Autodesk Inventor part; units mm, degrees
ref_plane "YZ Plane" through (0, 0, 0) normal (1, 0, 0) x (0, 1, 0)
ref_plane "XZ Plane" through (0, 0, 0) normal (0, 1, 0) x (-1, 0, 0)
ref_plane "XY Plane" through (0, 0, 0) normal (0, 0, 1) x (1, 0, 0)
sketch "Sketch1" plane through (0, 0, 0) normal (0, 0, 1) x (1, 0, 0)
  line L0 (0, 0) -> (35, 0)
  line L1 (35, 0) -> (35, 12)
  line L2 (0, 12) -> (0, 0)
  line L3 (0, 12) -> (-0.0372, 12)
  line L4 (35.0398, 12) -> (35, 12)
  line L5 (-0.0372, 12) -> (-0.0372, 30)
  line L6 (35.0398, 12) -> (35.0398, 30)
  arc A0 (35.0398, 30) -> (-0.0372, 30) centre (17.5013, 30) ccw
  circle A1 centre (17.5013, 30) radius 2
  dimension "d0" = 35
  dimension "d1" = 12
  dimension "d4" = 18
  dimension "d6" = 4
extrude "Extrusion1" add sketch "Sketch1" along normal blind 22.5
sketch "Sketch2" plane through (0, 0, 22.5) normal (0, 0, 1) x (1, 0, 0)
  line L0 (0, 2) -> (35, 2)
  line L1 (35, 2) -> (35, 10)
  line L2 (35, 10) -> (0, 10)
  line L3 (0, 10) -> (0, 2)
  point P0 (0, 0)
extrude "Extrusion2" cut sketch "Sketch2" against normal blind 20
sketch "Sketch3" plane through (-0.0372, 12, 0) normal (-1, 0, 0) x (0, 0, 1)
  point P0 (0, -12)
ref_plane "Work Plane1" through (17.5013, 47.5385, 0) normal (0, -1, 0) x (1, 0, 0)
sketch "Sketch4" plane through (17.5013, 47.5385, 0) normal (0, -1, 0) x (1, 0, 0)
  line L0 (17.5385, 0) -> (17.5385, 22.5)
  line L1 (-17.5385, 0) -> (-17.5385, 22.5)
  line L2 (17.5385, 20.5) -> (-17.5385, 20.5)
  line L3 (-17.5385, 20.5) -> (-17.5385, 2)
  line L4 (-17.5385, 2) -> (17.5385, 2)
  line L5 (17.5385, 2) -> (17.5385, 20.5)
  line L6 (17.5385, 22.5) -> (-17.5385, 22.5)
  point P0 (-17.5013, 0)
  dimension "d11" = 18.5
  dimension "d12" = 2
extrude "Extrusion3" cut sketch "Sketch4" along normal blind 35.5 contours L4 L1 L2 L0
properties part number "Maintients poullies V4"
The listing builds one solid part. Answer for the finished solid, in the listing's coordinates (mm). A direction names the side the tool comes from. Give positions to 0.01 mm unless a question says otherwise; leave off trailing zeros. Write each loop counter-clockwise with the first axis right and the second up, starting at its lowest first coordinate (ties: lowest second). Pieces come first, ordered by that corner, then holes. Notation, with made-up numbers: (-1, -31) - (42, -31) arc R31 ccw to (42, -3) - close; hole circle Ø3 at (49, 62.25). An arc over 180 degrees is marked (long way). One line per question, with ' | ' between items. Start each with the question number.
1. Given P1, Ø5.5, axis at x = 21, z = 14, coming from the +Y side; P2, Ø6, axis at y = 7.5, z = 14, coming from the -X side; P3, Ø2.5, axis at x = 24.5, y = 7.5, coming from the +Z side; P4, Ø3.5, axis at x = 17.5, y = 30, coming from the -Z side, each flat-ended and moving along its own axis, determine where each tip first touches the part or whether it passes through.
2. Determine the mould class of faces 6 (the face through (18.424, 31.774, 21.486)), 7 (the face through (17, 0, 11)), 8 (the face through (17, 6, 2.5)), 9 (the face through (-0.037, 20, 21)) for opening direction Y: +Y half, -Y half, draft (parallel to the pull), parting line (faces both ways), or undercut.
3. Section D-D, the plane x = 24 is taken. Determine the outline of the cut face in (y, z), then the cut area to 3 significant figures.
4. Section B-B, the plane x = 7.5 is taken. Determine the outline of the cut face in (y, z), then the cut area to 3 significant figures.
5. For faces 1 (the face through (17.116, 47.534, 0.986)), 2 (the face through (35, 1, 9)), 3 (the face through (18, 26, 20.5)), 4 (the face through (35.04, 20, 21)), 5 (the face through (17, 2, 13)), determine the directions among +Z, -Z, +X, -X, +Y, -Y from which every point of the face is accessible in a straight line to the end or side of a thin tool.
6. Section A-A, the plane y = 20 is taken. Determine the outline of the cut face in (x, z), then the cut area to 3 significant figures.
7. Section C-C, the plane y = 44 is taken. Determine the outline of the cut face in (x, z).
8. Straight lines are drawn through the part: line 1 (Y direction, x = 19.5, z = 20); line 2 (Z direction, x = 32.5, y = 21.5); line 3 (X direction, y = 30, z = 20.9). For each, find the intervals that lie inside material, in ascending order.
Result:
1) P1: stops at y = 12.04 | P2: stops at x = 0 | P3: stops at z = 2.5 | P4: passes through
2) face 6: undercut | face 7: -Y half | face 8: undercut | face 9: draft
3) outline: (0, 0) - (46.29, 0) - (46.29, 2) - (12.04, 2) - (12.04, 20.5) - (46.29, 20.5) - (46.29, 22.5) - (10, 22.5) - (10, 2.5) - (2, 2.5) - (2, 22.5) - (0, 22.5) - close | area: 248 mm2
4) outline: (0, 0) - (44.41, 0) - (44.41, 2) - (12.04, 2) - (12.04, 20.5) - (44.41, 20.5) - (44.41, 22.5) - (10, 22.5) - (10, 2.5) - (2, 2.5) - (2, 22.5) - (0, 22.5) - close | area: 240 mm2
5) face 1: +Z, -Z, +Y | face 2: +Z, -Z, +X, -Y | face 3: +X, -X, +Y | face 4: +Z, -Z, +X, +Y, -Y | face 5: +Z, +X, -X
6) outline: (-0.04, 0) - (35.04, 0) - (35.04, 2) - (-0.04, 2) - close; (-0.04, 20.5) - (35.04, 20.5) - (35.04, 22.5) - (-0.04, 22.5) - close | area: 140 mm2
7) outline: (6.94, 0) - (28.07, 0) - (28.07, 2) - (6.94, 2) - close; (6.94, 20.5) - (28.07, 20.5) - (28.07, 22.5) - (6.94, 22.5) - close
8) line 1: y = 0 to 2, 10 to 12.04 | line 2: z = 0 to 2, 20.5 to 22.5 | line 3: x = -0.04 to 15.5, 19.5 to 35.04
